For this review, take the finished solid that the model builds, in its own axes (mm). Face numbers are marked on the shaded views. Round coordinates to 2 decimals unless told otherwise and drop trailing zeros. Loops run counter-clockwise (first coordinate to the right, second up) from the corner with the lowest first, then second, coordinate; pieces in that order, holes last.
1) Insertion check: pin 1 (1 mm diameter, centred on y = 16, z = -27.5, fed in from +X); pin 2 (1.5 mm diameter, centred on y = 14, z = -27, fed in from +X); pin 3 (3 mm diameter, centred on x = 0, z = -31.75, fed in from -Y). Each pin has a flat end and moves straight along its axis. Give the tip position at first contact, or say it passes through.
2) Take a section at D-D (z = 31.75). State the section outline as (x, y) points.
3) Take a section at B-B (y = 9). State the section outline as (x, z) points.
4) Take a section at A-A (z = 8). State the section outline as (x, y) points.
5) Take a section at C-C (x = 0). State the section outline as (y, z) points (3 decimals).
6) Wall thickness on L1, parallel to Z at x = 0, y = 5.4 (3 decimals); L2, parallel to Y at x = -0.25, z = 10; L3, parallel to X at y = 15.25, z = 32: over which ranges is each line inside the solid? List them lowest first.
7) Mouldability with a two-part tool opening along Y and no side actions: class the marked faces 1, 2 and 3 as pulls with the +Y half, pulls with the -Y half, needs draft (parallel to the pull), parting line crosses it, or undercut.
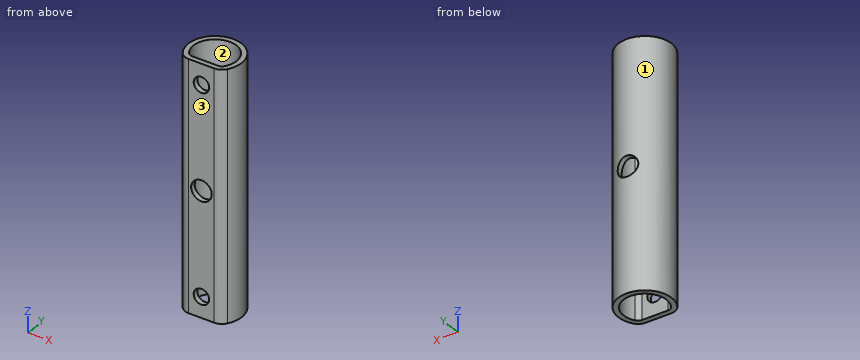
```python
from build123d import *

# Parameters (mm, degrees)
BOSS_EXTRUDE1_DEPTH      = 76.2
CUT_EXTRUDE1_DEPTH       = 77.2
M4_CLEARANCE_HOLE1_D     = 4.7752
M4_CLEARANCE_HOLE1_DEPTH = 1.5875
HOLE1_D                  = 6.35
HOLE1_DEPTH              = 14.2494
FILLET1_R                = 1.9304
FILLET2_R                = 3.5179


with BuildPart() as part:
    # Sketch1 → Boss-Extrude1 (new body)
    with BuildSketch(Plane(origin=(0, 0, -38.1), x_dir=(-1, 0, 0), z_dir=(0, 0, -1))):
        with BuildLine():
            Line((-5.533344062, 4.9784), (5.533344062, 4.9784))
            ThreePointArc((5.533344062, 4.9784), (0, 19.2278), (-5.533344062, 4.9784))
        make_face()
    extrude(amount=-BOSS_EXTRUDE1_DEPTH)

    # Sketch2 → Cut-Extrude1 (cut, through all)
    with BuildSketch(Plane.XY.offset(38.1)):
        with BuildLine():
            Line((-4.878086413, 6.5659), (4.878086413, 6.5659))
            ThreePointArc((4.878086413, 6.5659), (0, 17.6403), (-4.878086413, 6.5659))
        make_face()
    extrude(amount=-CUT_EXTRUDE1_DEPTH, mode=Mode.SUBTRACT)

    # M4 Clearance Hole1
    with Locations(Plane(origin=(0, 4.9784, 0), x_dir=(-1, 0, 0), z_dir=(0, -1, 0))):
        with Locations((0, 0), (0, 31.75), (0, -31.75)):
            Hole(M4_CLEARANCE_HOLE1_D / 2, depth=M4_CLEARANCE_HOLE1_DEPTH)

    # Hole1
    with Locations(Plane(origin=(0, 19.2278, 0), x_dir=(1, 0, 0), z_dir=(0, 1, 0))):
        with Locations((0, 0)):
            Hole(HOLE1_D / 2, depth=HOLE1_DEPTH)

    # Fillet1
    fillet1_edges = [part.edges().sort_by_distance(p)[0] for p in [
        (-4.878086413, 6.5659, 0),
        (4.878086413, 6.5659, 0),
    ]]
    fillet(fillet1_edges, radius=FILLET1_R)

    # Fillet2
    fillet2_edges = [part.edges().sort_by_distance(p)[0] for p in [
        (-5.533344062, 4.9784, 0),
        (5.533344062, 4.9784, 0),
    ]]
    fillet(fillet2_edges, radius=FILLET2_R)


solid = part.part
```
Response:
1. pin 1: stops at x = 6.87
1. pin 2: stops at x = 7.89
1. pin 3: stops at y = 17.47
2. outline: (-6.9, 6.59) arc R3.52 ccw to (-3.94, 4.98) - (-2.39, 4.98) - (-2.39, 6.57) - (-3.94, 6.57) arc R1.93 cw to (-5.56, 7.45) arc R6.61 cw (long way) to (5.56, 7.45) arc R1.93 cw to (3.94, 6.57) - (2.39, 6.57) - (2.39, 4.98) - (3.94, 4.98) arc R3.52 ccw to (6.9, 6.59) arc R8.2 ccw (long way) to start
3. outline: (-7.94, -38.1) - (-6.29, -38.1) - (-6.29, 38.1) - (-7.94, 38.1) - close; (6.29, -38.1) - (7.94, -38.1) - (7.94, 38.1) - (6.29, 38.1) - close
4. outline: (-6.9, 6.59) arc R3.52 ccw to (-3.94, 4.98) - (3.94, 4.98) arc R3.52 ccw to (6.9, 6.59) arc R8.2 ccw (long way) to start; hole (-5.56, 7.45) arc R1.93 ccw to (-3.94, 6.57) - (3.94, 6.57) arc R1.93 ccw to (5.56, 7.45) arc R6.61 ccw (long way) to start
5. outline: (4.978, -38.1) - (6.566, -38.1) - (6.566, -34.138) - (4.978, -34.138) - close; (4.978, -29.362) - (6.566, -29.362) - (6.566, -3.175) - (4.978, -3.175) - close; (4.978, 3.175) - (6.566, 3.175) - (6.566, 29.362) - (4.978, 29.362) - close; (4.978, 34.138) - (6.566, 34.138) - (6.566, 38.1) - (4.978, 38.1) - close; (17.64, -38.1) - (19.228, -38.1) - (19.228, -3.175) - (17.64, -3.175) - close; (17.64, 3.175) - (19.228, 3.175) - (19.228, 38.1) - (17.64, 38.1) - close
6. L1: z = -38.1 to -34.138, -29.362 to -3.175, 3.175 to 29.362, 34.138 to 38.1
6. L2: y = 4.98 to 6.57, 17.64 to 19.22
6. L3: x = -7.03 to -5.09, 5.09 to 7.03
7. face 1: parting line crosses it
7. face 2: undercut
7. face 3: pulls with the -Y half
